Design review of the part built by this model. Coordinates are the model's own, in mm. Coordinates: 2 decimals unless noted, no trailing zeros. Loops run counter-clockwise (first coordinate to the right, second up) from the corner with the lowest first, then second, coordinate; pieces in that order, holes last. Notation, with made-up numbers: (-31, -28) - (23, -28) arc R23 cw to (23, -17) - close; hole circle Ø7 at (51, 23). An arc over 180 degrees is marked (long way). Answer in a Markdown table with one row per item. Add a question column.
(1) We need section A-A, the plane x = -6. Write out the cut boundary in (y, z).
(2) The part is to be moulded in two halves that separate along Y. For faces 1 (the face through (-5.26, -9.24, 3.55)), 2 (the face through (-7, 11, 3)), 3 (the face through (-10.76, -6.13, 3.55)), say which applies: released by +Y, released by -Y, zero draft, split by the parting line, or undercut.
(3) We need section C-C, the plane z = 1. Write out the cut boundary in (x, y), plus the area to 3 significant figures.
(4) To check wall thickness, follow L1, parallel to Y at x = 6.5, z = 6.5; L2, parallel to Y at x = -6, z = 3.5; L3, parallel to X at y = 5, z = 6.5. State the ranges of each line that lie inside material, in increasing order. Write a range as [from, to].
(5) We need section B-B, the plane y = -2. Write out the cut boundary in (x, z).
(6) We need section D-D, the plane y = 7. Write out the cut boundary in (x, z), plus the area to 3 significant figures.
from build123d import *

# Parameters (mm, degrees)
F0_W     = 23
F0_H     = 25
F1_DEPTH = 7
F3_DEPTH = 25.001
F4_DEPTH = 12.5
F5_SIZE  = 6
F6_R     = 10
F7_R     = 1.6
F8_DEPTH = 25


with BuildPart() as f1:
    # F0 (on Top) → F1 (new body)
    with BuildSketch(Plane.XY):
        Rectangle(F0_W, F0_H)
    extrude(amount=F1_DEPTH)

    # F2 (on face) → F3 (cut, through all)
    with BuildSketch(Plane.XZ.offset(12.5)):
        with BuildLine():
            Line((0, 7), (-2.2912878475, 7))
            ThreePointArc((-2.2912878475, 7), (0, 5.5), (2.2912878475, 7))
            Line((2.2912878475, 7), (0, 7))
        make_face()
    extrude(amount=-F3_DEPTH, mode=Mode.SUBTRACT)

    # F2 (on face) → F4 (cut)
    with BuildSketch(Plane.XZ.offset(12.5)):
        with BuildLine():
            ThreePointArc((2.2912878475, 7), (0, 5.5), (-2.2912878475, 7))
            Line((-2.2912878475, 7), (-2.8084005449, 7))
            Line((-2.8084005449, 7), (-3.0722061624, 6.9397880893))
            ThreePointArc((-3.0722061624, 6.9397880893), (-2.9281488207, 6.5898778479), (-2.7443962613, 6.2590838157))
            Line((-2.7443962613, 6.2590838157), (-2.4464411557, 6.4966950836))
            Line((-2.4464411557, 6.4966950836), (-2.0099982944, 5.9494130458))
            Line((-2.0099982944, 5.9494130458), (-2.3079534, 5.711801778))
            ThreePointArc((-2.3079534, 5.711801778), (-2.026341856, 5.459047682), (-1.7172603691, 5.2407398048))
            Line((-1.7172603691, 5.2407398048), (-1.5519077603, 5.5840980352))
            Line((-1.5519077603, 5.5840980352), (-0.9212295527, 5.2803794178))
            Line((-0.9212295527, 5.2803794178), (-1.0865821616, 4.9370211875))
            ThreePointArc((-1.0865821616, 4.9370211875), (-0.7231930354, 4.8314842854), (-0.35, 4.7689011157))
            Line((-0.35, 4.7689011157), (-0.35, 5.15))
            Line((-0.35, 5.15), (0.35, 5.15))
            Line((0.35, 5.15), (0.35, 4.7689011157))
            ThreePointArc((0.35, 4.7689011157), (0.7231930354, 4.8314842854), (1.0865821616, 4.9370211875))
            Line((1.0865821616, 4.9370211875), (0.9212295527, 5.2803794178))
            Line((0.9212295527, 5.2803794178), (1.5519077603, 5.5840980352))
            Line((1.5519077603, 5.5840980352), (1.7172603691, 5.2407398048))
            ThreePointArc((1.7172603691, 5.2407398048), (2.026341856, 5.459047682), (2.3079534, 5.711801778))
            Line((2.3079534, 5.711801778), (2.0099982944, 5.9494130458))
            Line((2.0099982944, 5.9494130458), (2.4464411557, 6.4966950836))
            Line((2.4464411557, 6.4966950836), (2.7443962613, 6.2590838157))
            ThreePointArc((2.7443962613, 6.2590838157), (2.9281488207, 6.5898778479), (3.0722061624, 6.9397880893))
            Line((3.0722061624, 6.9397880893), (2.8084005449, 7))
            Line((2.8084005449, 7), (2.2912878475, 7))
        make_face()
        with BuildLine():
            Line((3.0719063417, 5.9979032421), (2.7443962613, 6.2590838157))
            ThreePointArc((2.7443962613, 6.2590838157), (2.540952318, 5.973658144), (2.3079534, 5.711801778))
            Line((2.3079534, 5.711801778), (2.6354634804, 5.4506212044))
            Line((2.6354634804, 5.4506212044), (3.0719063417, 5.9979032421))
        make_face()
        with BuildLine():
            ThreePointArc((2.3079534, 5.711801778), (2.540952318, 5.973658144), (2.7443962613, 6.2590838157))
            Line((2.7443962613, 6.2590838157), (2.4464411557, 6.4966950836))
            Line((2.4464411557, 6.4966950836), (2.0099982944, 5.9494130458))
            Line((2.0099982944, 5.9494130458), (2.3079534, 5.711801778))
        make_face()
        with BuildLine():
            Line((1.8990147515, 4.8633229408), (1.7172603691, 5.2407398048))
            ThreePointArc((1.7172603691, 5.2407398048), (1.4101221521, 5.0718511793), (1.0865821616, 4.9370211875))
            Line((1.0865821616, 4.9370211875), (1.268336544, 4.5596043235))
            Line((1.268336544, 4.5596043235), (1.8990147515, 4.8633229408))
        make_face()
        with BuildLine():
            ThreePointArc((1.0865821616, 4.9370211875), (1.4101221521, 5.0718511793), (1.7172603691, 5.2407398048))
            Line((1.7172603691, 5.2407398048), (1.5519077603, 5.5840980352))
            Line((1.5519077603, 5.5840980352), (0.9212295527, 5.2803794178))
            Line((0.9212295527, 5.2803794178), (1.0865821616, 4.9370211875))
        make_face()
        with BuildLine():
            ThreePointArc((0.35, 4.7689011157), (0, 4.75), (-0.35, 4.7689011157))
            Line((-0.35, 4.7689011157), (-0.35, 4.35))
            Line((-0.35, 4.35), (0.35, 4.35))
            Line((0.35, 4.35), (0.35, 4.7689011157))
        make_face()
        with BuildLine():
            Line((-0.35, 5.15), (-0.35, 4.7689011157))
            ThreePointArc((-0.35, 4.7689011157), (0, 4.75), (0.35, 4.7689011157))
            Line((0.35, 4.7689011157), (0.35, 5.15))
            Line((0.35, 5.15), (-0.35, 5.15))
        make_face()
        with BuildLine():
            ThreePointArc((-1.0865821616, 4.9370211875), (-1.4101221521, 5.0718511793), (-1.7172603691, 5.2407398048))
            Line((-1.7172603691, 5.2407398048), (-1.8990147515, 4.8633229408))
            Line((-1.8990147515, 4.8633229408), (-1.268336544, 4.5596043235))
            Line((-1.268336544, 4.5596043235), (-1.0865821616, 4.9370211875))
        make_face()
        with BuildLine():
            Line((-1.5519077603, 5.5840980352), (-1.7172603691, 5.2407398048))
            ThreePointArc((-1.7172603691, 5.2407398048), (-1.4101221521, 5.0718511793), (-1.0865821616, 4.9370211875))
            Line((-1.0865821616, 4.9370211875), (-0.9212295527, 5.2803794178))
            Line((-0.9212295527, 5.2803794178), (-1.5519077603, 5.5840980352))
        make_face()
        with BuildLine():
            ThreePointArc((-2.3079534, 5.711801778), (-2.540952318, 5.973658144), (-2.7443962613, 6.2590838157))
            Line((-2.7443962613, 6.2590838157), (-3.0719063417, 5.9979032421))
            Line((-3.0719063417, 5.9979032421), (-2.6354634804, 5.4506212044))
            Line((-2.6354634804, 5.4506212044), (-2.3079534, 5.711801778))
        make_face()
        with BuildLine():
            Line((-2.4464411557, 6.4966950836), (-2.7443962613, 6.2590838157))
            ThreePointArc((-2.7443962613, 6.2590838157), (-2.540952318, 5.973658144), (-2.3079534, 5.711801778))
            Line((-2.3079534, 5.711801778), (-2.0099982944, 5.9494130458))
            Line((-2.0099982944, 5.9494130458), (-2.4464411557, 6.4966950836))
        make_face()
        with BuildLine():
            Line((3.0923292192, 7), (2.8084005449, 7))
            Line((2.8084005449, 7), (3.0722061624, 6.9397880893))
            ThreePointArc((3.0722061624, 6.9397880893), (3.0824147168, 6.969844908), (3.0923292192, 7))
        make_face()
        with BuildLine():
            Line((-3.0722061624, 6.9397880893), (-2.8084005449, 7))
            Line((-2.8084005449, 7), (-3.0923292192, 7))
            ThreePointArc((-3.0923292192, 7), (-3.0824147168, 6.969844908), (-3.0722061624, 6.9397880893))
        make_face()
    extrude(amount=-F4_DEPTH, mode=Mode.SUBTRACT)

    # F5
    f5_edges = [f1.edges().sort_by_distance(p)[0] for p in [
        (11.5, -12.5, 3.5),
        (-11.5, -12.5, 3.5),
        (11.5, 12.5, 3.5),
        (-11.5, 12.5, 3.5),
    ]]
    chamfer(f5_edges, length=F5_SIZE)

    # F6
    f6_edges = [f1.edges().sort_by_distance(p)[0] for p in [
        (11.5, 6.5, 3.5),
        (11.5, -6.5, 3.5),
        (-11.5, 6.5, 3.5),
        (-11.5, -6.5, 3.5),
    ]]
    fillet(f6_edges, radius=F6_R)

    # F7 (on face) → F8 (cut)
    with BuildSketch(Plane.XY.offset(7)):
        with Locations((6, -7.8212832158)):
            Circle(F7_R)
        with Locations((-6, -7.8212832158)):
            Circle(F7_R)
        with Locations((-6, 7.8212832158)):
            Circle(F7_R)
        with Locations((6, 7.8212832158)):
            Circle(F7_R)
    extrude(amount=-F8_DEPTH, mode=Mode.SUBTRACT)


solid = f1.part
Responses:
| question | item | result |
|---|---|---|
| 1 | outline | (-12, 0) - (-9.42, 0) - (-9.42, 7) - (-12, 7) - close; (-6.22, 0) - (6.22, 0) - (6.22, 7) - (-6.22, 7) - close; (9.42, 0) - (12, 0) - (12, 7) - (9.42, 7) - close |
| 2 | face 1 | undercut |
| 2 | face 2 | released by +Y |
| 2 | face 3 | released by -Y |
| 3 | outline | (-11.5, -2.36) arc R10 ccw to (-8.57, -9.43) - (-5.5, -12.5) - (5.5, -12.5) - (8.57, -9.43) arc R10 ccw to (11.5, -2.36) - (11.5, 2.36) arc R10 ccw to (8.57, 9.43) - (5.5, 12.5) - (-5.5, 12.5) - (-8.57, 9.43) arc R10 ccw to (-11.5, 2.36) - close; hole circle Ø3.2 at (-6, -7.82); hole circle Ø3.2 at (-6, 7.82); hole circle Ø3.2 at (6, -7.82); hole circle Ø3.2 at (6, 7.82) |
| 3 | area | 462 mm2 |
| 4 | L1 | y = [-11.5, -9.34], [-6.3, 6.3], [9.34, 11.5] |
| 4 | L2 | y = [-12, -9.42], [-6.22, 6.22], [9.42, 12] |
| 4 | L3 | x = [-11.14, -2], [2, 11.14] |
| 5 | outline | (-11.5, 0) - (11.5, 0) - (11.5, 7) - (3.09, 7) arc R3.25 cw to (2.74, 6.26) - (3.07, 6) - (2.64, 5.45) - (2.31, 5.71) arc R3.25 cw to (1.72, 5.24) - (1.9, 4.86) - (1.27, 4.56) - (1.09, 4.94) arc R3.25 cw to (0.35, 4.77) - (0.35, 4.35) - (-0.35, 4.35) - (-0.35, 4.77) arc R3.25 cw to (-1.09, 4.94) - (-1.27, 4.56) - (-1.9, 4.86) - (-1.72, 5.24) arc R3.25 cw to (-2.31, 5.71) - (-2.64, 5.45) - (-3.07, 6) - (-2.74, 6.26) arc R3.25 cw to (-3.09, 7) - (-11.5, 7) - close |
| 6 | outline | (-10.36, 0) - (-7.37, 0) - (-7.37, 7) - (-10.36, 7) - close; (-4.63, 0) - (4.63, 0) - (4.63, 7) - (2.29, 7) arc R2.5 cw to (-2.29, 7) - (-4.63, 7) - close; (7.37, 0) - (10.36, 0) - (10.36, 7) - (7.37, 7) - close |
| 6 | area | 102 mm2 |
